from build123d import *

# Parameters (mm, degrees)
CYLINDER002_R     = 0.6
CYLINDER002_DEPTH = 4
CYLINDER001_R     = 6
CYLINDER001_DEPTH = 6
CYLINDER_R        = 4
CYLINDER_DEPTH    = 6
CUBE004_W         = 6.025
CUBE004_H         = 3.95
CUBE004_DEPTH     = 4
CUBE003_W         = 6.025
CUBE003_H         = 3.95
CUBE003_DEPTH     = 4
CUBE002_W         = 15.25
CUBE002_H         = 11.6
CUBE002_DEPTH     = 4
CUBE001_W         = 15.25
CUBE001_H         = 3.95
CUBE001_DEPTH     = 4
CUBE_W            = 13.25
CUBE_H            = 11.6
CUBE_DEPTH        = 4


with BuildPart() as cylinder002:
    # cylinder002 → cylinder002 (new body)
    with BuildSketch(Plane(origin=(6.625, -10, -1), x_dir=(1, 0, 0), z_dir=(0, 0, 1))):
        Circle(CYLINDER002_R)
    extrude(amount=CYLINDER002_DEPTH)


with BuildPart() as cylinder001:
    # cylinder001 → cylinder001 (new body)
    with BuildSketch(Plane(origin=(16.25, 0, 0), x_dir=(1, 0, 0), z_dir=(0, 0, 1))):
        Circle(CYLINDER001_R)
    extrude(amount=CYLINDER001_DEPTH)


with BuildPart() as cylinder:
    # cylinder → cylinder (new body)
    with BuildSketch(Plane.XY):
        Circle(CYLINDER_R)
    extrude(amount=CYLINDER_DEPTH)


with BuildPart() as cube004:
    # cube004 → cube004 (new body)
    with BuildSketch(Plane(origin=(8.225, -12.6, -1), x_dir=(1, 0, 0), z_dir=(0, 0, 1))):
        with Locations((3.0125, 1.975)):
            Rectangle(CUBE004_W, CUBE004_H)
    extrude(amount=CUBE004_DEPTH)


with BuildPart() as cube003:
    # cube003 → cube003 (new body)
    with BuildSketch(Plane(origin=(-1, -12.6, -1), x_dir=(1, 0, 0), z_dir=(0, 0, 1))):
        with Locations((3.0125, 1.975)):
            Rectangle(CUBE003_W, CUBE003_H)
    extrude(amount=CUBE003_DEPTH)


with BuildPart() as cube002:
    # cube002 → cube002 (new body)
    with BuildSketch(Plane(origin=(-1, -8.4, -0.25), x_dir=(1, 0, 0), z_dir=(0, 0, 1))):
        with Locations((7.625, 5.8)):
            Rectangle(CUBE002_W, CUBE002_H)
    extrude(amount=CUBE002_DEPTH)


with BuildPart() as cube001:
    # cube001 → cube001 (new body)
    with BuildSketch(Plane(origin=(-1, -1, 0.25), x_dir=(1, 0, 0), z_dir=(0, 0, 1))):
        with Locations((7.625, 1.975)):
            Rectangle(CUBE001_W, CUBE001_H)
    extrude(amount=CUBE001_DEPTH)


with BuildPart() as difference006:
    # cube → cube (new body)
    with BuildSketch(Plane.XY):
        with Locations((6.625, 5.8)):
            Rectangle(CUBE_W, CUBE_H)
    extrude(amount=CUBE_DEPTH)

    # difference: cut cube001
    add(cube001.part, mode=Mode.SUBTRACT)


with BuildPart() as difference006_1:
    # difference placement: moved
    add(difference006.part.moved(Location((0, -11.6, 0))))

    # difference001: cut cube002
    add(cube002.part, mode=Mode.SUBTRACT)

    # difference002: cut cube003
    add(cube003.part, mode=Mode.SUBTRACT)

    # difference003: cut cube004
    add(cube004.part, mode=Mode.SUBTRACT)

    # difference004: cut cylinder
    add(cylinder.part, mode=Mode.SUBTRACT)

    # difference005: cut cylinder001
    add(cylinder001.part, mode=Mode.SUBTRACT)

    # difference006: cut cylinder002
    add(cylinder002.part, mode=Mode.SUBTRACT)


solid = difference006_1.part
Check sheet for the modelled part. Datum: model origin and axes. Units: mm. A direction names the side the tool comes from. Coordinates: 2 decimals unless noted, no trailing zeros. Write each loop counter-clockwise with the first axis right and the second up, starting at its lowest first coordinate (ties: lowest second). Pieces come first, ordered by that corner, then holes. Notation, with made-up numbers: M 39,12.5 L 59,12.5 A16 ccw 59,42.5 Z; hole C 20.5,13 d6. An arc over 180 degrees is marked long. Answer as CSV lines item,"result".
Q1. Cross-section at D-D (z = 3.5). Record the boundary of the cut face in (x, y).
Check result:
outline,"M 0,-8.65 L 13.25,-8.65 L 13.25,-8.4 L 0,-8.4 Z"
Q2. Set-up check for faces 1 (the face through (7, -11, 0.25)), 2 (the face through (7, -8.4, 2)), 3 (the face through (7, -9, 0)): record each of +Z, -Z, +X, -X, +Y, -Y from which the full face is reachable in a straight line by a thin tool's end or side.
Check result:
face 1,"+Z, +X, -X, -Y"
face 2,"-Z, +X, -X, +Y"
face 3,"-Z, +X, -X, +Y, -Y"
Q3. Cross-section at A-A (y = -10). Record the boundary of the cut face in (x, z) (3 decimals), then the cut area to 3 significant figures.
Check result:
outline,"M 5.025,0 L 6.025,0 L 6.025,0.25 L 5.025,0.25 Z; M 7.225,0 L 8.225,0 L 8.225,0.25 L 7.225,0.25 Z"
area,"0.500 mm^2"
Q4. Cross-section at C-C (x = 9.25). Record the boundary of the cut face in (y, z), then the cut area to 3 significant figures.
Check result:
outline,"M -8.65,0 L -8.4,0 L -8.4,3.75 L 0,3.75 L 0,4 L -8.65,4 Z"
area,"3.10 mm^2"
Q5. Cross-section at B-B (x = 7). Record the boundary of the cut face in (y, z), then the cut area to 3 significant figures.
Check result:
outline,"M -11.6,0 L -10.47,0 L -10.47,0.25 L -11.6,0.25 Z; M -9.53,0 L -8.4,0 L -8.4,3.75 L 0,3.75 L 0,4 L -8.65,4 L -8.65,0.25 L -9.53,0.25 Z"
area,"3.60 mm^2"
Q6. Go/stop test with flat-tipped pins: pin 1 (6.5 mm diameter, centred on x = 4, y = -4, fed in from -Z); pin 2 (0.9 mm diameter, centred on x = 6.5, y = -9.5, fed in from +Z). Record where each tip stops, or that it passes through.
Check result:
pin 1,"z = 3.75"
pin 2,"z = 0.25"
Q7. Material ranges on probe 1 along X at (y, z) = (-10, 0.15) (3 decimals); probe 2 along Y at (x, z) = (4, 2.45); probe 3 along Z at (x, y) = (3, -6), recorded low to high. Write a range as from..to.
Check result:
probe 1,"5.025..6.025, 7.225..8.225"
probe 2,"-8.65..-8.4"
probe 3,"3.75..4"
